Here's the drawing with two shaded views (mm, measured from the low corner). I have some questions. Coordinates: 2 decimals unless noted, no trailing zeros. Order: outer loops, then holes, each group sorted by start corner. A loop starts at its lowest first (then second) coordinate and runs counter-clockwise, first axis right, second up. Notation, with made-up numbers: (57.5, -6) -> (63.5, -6) arc R25 ccw to (63.5, 11) -> close; hole circle Ø2 at (51.25, 82). An arc over 180 degrees is marked (long way). Answer as a JSON object with one key per item and string values. Group by question number.
(1) I need wall thicknesses on line 1 (X direction, y = 25.4, z = 10.25) (1 decimal); line 2 (Y direction, x = 105.5, z = 3.5); line 3 (Y direction, x = 262.5, z = 4.5). Which ranges of each line are inside material? Lowest first, please.
(2) I want a section at C-C, the plane x = 330.2. List the corners of the cut face in (y, z) for me.
(3) I want a section at A-A, the plane y = 101.6. List the corners of the cut face in (x, z) for me.
(4) I want a section at B-B, the plane z = 6.25. List the corners of the cut face in (x, y) for me, plus the area to 3 significant figures.
(5) For pin 1 (4 mm diameter, centred on y = 115.5, z = 8, fed in from -X); pin 2 (11 mm diameter, centred on x = 330.2, y = 101.6, fed in from -Z); pin 3 (1 mm diameter, centred on x = 233.5, z = 8.5, fed in from +Y) (1 decimal), each with a flat end and sliding along its axis, tell me the tip position at first contact or that it passes through.
(6) I want a section at D-D, the plane x = 288.5. List the corners of the cut face in (y, z) for me.
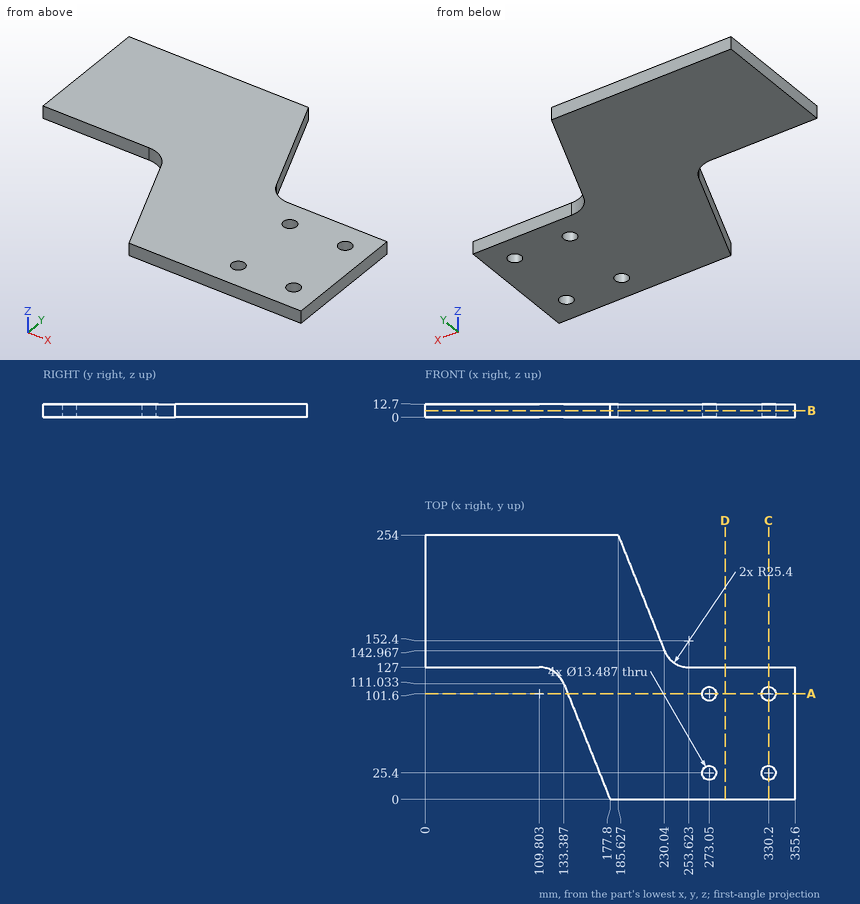
Computed values:
{
 "1": {"line 1": "x = 167.6 to 266.3, 279.8 to 323.5, 336.9 to 355.6", "line 2": "y = 127 to 254", "line 3": "y = 0 to 127"},
 "2": {"outline": "(0, 0) -> (18.66, 0) -> (18.66, 12.7) -> (0, 12.7) -> close; (32.14, 0) -> (94.86, 0) -> (94.86, 12.7) -> (32.14, 12.7) -> close; (108.34, 0) -> (127, 0) -> (127, 12.7) -> (108.34, 12.7) -> close"},
 "3": {"outline": "(137.16, 0) -> (266.31, 0) -> (266.31, 12.7) -> (137.16, 12.7) -> close; (279.79, 0) -> (323.46, 0) -> (323.46, 12.7) -> (279.79, 12.7) -> close; (336.94, 0) -> (355.6, 0) -> (355.6, 12.7) -> (336.94, 12.7) -> close"},
 "4": {"outline": "(0, 127) -> (109.8, 127) arc R25.4 cw to (133.39, 111.03) -> (177.8, 0) -> (355.6, 0) -> (355.6, 127) -> (253.62, 127) arc R25.4 cw to (230.04, 142.97) -> (185.63, 254) -> (0, 254) -> close; hole circle Ø13.49 at (273.05, 25.4); hole circle Ø13.49 at (273.05, 101.6); hole circle Ø13.49 at (330.2, 25.4); hole circle Ø13.49 at (330.2, 101.6)", "area": "52,100 mm2"},
 "5": {"pin 1": "stops at x = 129.61", "pin 2": "passes through", "pin 3": "stops at y = 137.6"},
 "6": {"outline": "(0, 0) -> (127, 0) -> (127, 12.7) -> (0, 12.7) -> close"}
}
